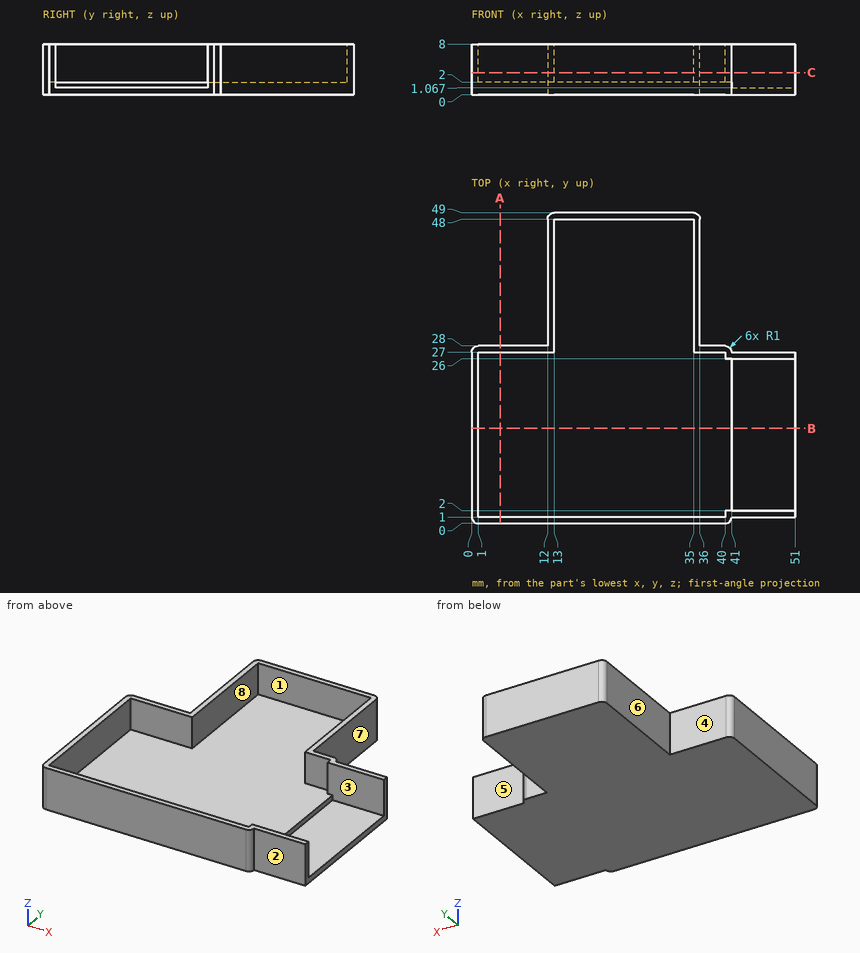
Drawing for the job (mm, zero at the part's lowest x, y, z). A direction names the side the tool comes from. Give positions to 0.01 mm unless a question says otherwise; leave off trailing zeros. Loops run counter-clockwise (first coordinate to the right, second up) from the corner with the lowest first, then second, coordinate; pieces in that order, holes last.
(1) Band-saw the part on A-A (x = 4.5). Write the cut outline in (y, z).
Return value:
outline: (0, 0) - (28, 0) - (28, 8) - (27, 8) - (27, 2) - (1, 2) - (1, 8) - (0, 8) - close
(2) Pin check, flat tips, straight feed: pin 1 (11 mm diameter, centred on x = 44.5, y = 19.5, fed in from +Z); pin 2 (1 mm diameter, centred on x = 45.5, z = 2, fed in from +Y); pin 3 (1.2 mm diameter, centred on x = 37, z = 2, fed in from +Y). Stop position of each tip, or through.
Return value:
pin 1: stops at z = 2
pin 2: stops at y = 27
pin 3: stops at y = 28
(3) Drill centre lines: line 1 along Y through (x, z) = (31.5, 6); line 2 along Y through (x, z) = (45, 3); line 3 along X through (y, z) = (32.5, 4). Where is each one in solid material? Low to high.
Return value:
line 1: y = 0 to 1, 48 to 49
line 2: y = 1 to 2, 26 to 27
line 3: x = 12 to 13, 35 to 36
(4) Band-saw the part on C-C (z = 3.5). Write the cut outline in (x, y), and give its area (3 significant figures).
Return value:
outline: (0, 1) arc R1 ccw to (1, 0) - (40, 0) arc R1 ccw to (41, 1) - (51, 1) - (51, 2) - (40, 2) - (40, 1) - (1, 1) - (1, 27) - (13, 27) - (13, 48) - (35, 48) - (35, 27) - (40, 27) - (40, 26) - (51, 26) - (51, 27) - (41, 27) arc R1 ccw to (40, 28) - (36, 28) - (36, 48) arc R1 ccw to (35, 49) - (13, 49) arc R1 ccw to (12, 48) - (12, 28) - (1, 28) arc R1 ccw to (0, 27) - close
area: 171 mm2
(5) 3-axis set-ups, long thin cutter, end or side, ignore diameter. For the marked faces 1, 2, 3 and 4: which of +Z, -Z, +X, -X, +Y, -Y reach the whole face in a straight line?
Return value:
face 1: +Z
face 2: +Z, -Z, +X, -Y
face 3: +Z, +X
face 4: +Z, -Z, -X, +Y
(6) Pull direction X, two halves, no side cores. Call the marked faces 5, 6, 7 and 8: pulls with the +X half, pulls with the -X half, needs draft (parallel to the pull), parting line crosses it, or undercut.
Return value:
face 5: needs draft
face 6: pulls with the -X half
face 7: pulls with the +X half
face 8: undercut
(7) Band-saw the part on B-B (y = 15). Write the cut outline in (x, z).
Return value:
outline: (0, 0) - (51, 0) - (51, 1.07) - (41, 1.07) - (41, 2) - (1, 2) - (1, 8) - (0, 8) - close
